```python
from build123d import *

# Parameters (mm, degrees)
F1_DEPTH = 13
F2_R     = 1
F3_DEPTH = 1.5
F4_R     = 2
F5_DEPTH = 3


with BuildPart() as f1:
    # F0 (on Top) → F1 (new body)
    with BuildSketch(Plane.XY):
        Polygon((-10.700272, 20.6891), (-33.300272, 20.6891), (-33.300272, 4.6891), (-38.300272, 4.6891), (-38.300272, 3.1891), (-33.300272, 3.1891), (-33.300272, -2.5109), (-10.700272, -2.5109), (-10.700272, 3.1891), (-5.700272, 3.1891), (-5.700272, 4.6891), (-10.700272, 4.6891), align=None)
    extrude(amount=F1_DEPTH)

    # F2 (on face) → F3 (cut, through all)
    with BuildSketch(Plane.XZ.offset(-3.1891)):
        with Locations((-36.300272, 6.5)):
            Circle(F2_R)
        with Locations((-7.700272, 6.5)):
            Circle(F2_R)
    extrude(amount=-F3_DEPTH, mode=Mode.SUBTRACT)

    # F4 (on face) → F5 (join)
    with BuildSketch(Plane.XZ.offset(2.5109)):
        with Locations((-16.700272, 6.5)):
            Circle(F4_R)
    extrude(amount=F5_DEPTH)


solid = f1.part
```
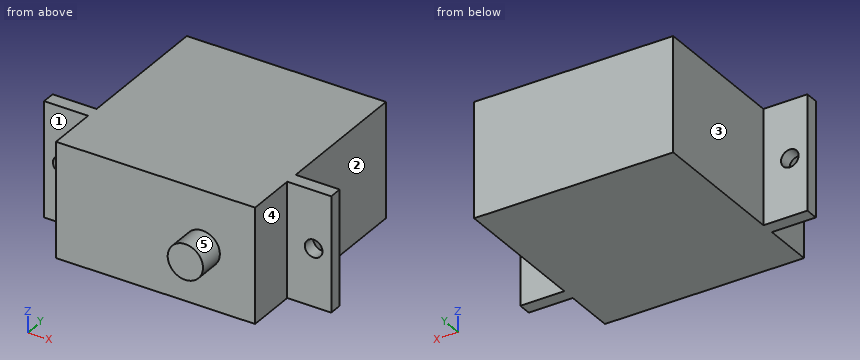
Could you check a few things on this model? Use its own coordinates, in mm. Face numbers are marked on the shaded views. A direction names the side the tool comes from. Round coordinates to 2 decimals unless told otherwise and drop trailing zeros. Loops run counter-clockwise (first coordinate to the right, second up) from the corner with the lowest first, then second, coordinate; pieces in that order, holes last. Notation, with made-up numbers: (15.5, -7.5) - (42.5, -7.5) arc R33 ccw to (42.5, 21.5) - close; hole circle Ø4 at (-38.75, -40). An arc over 180 degrees is marked (long way). Answer in a Markdown table with one row per item. Add a question column.
(1) I'm going to push flat-ended pins straight in: pin 1 (1 mm diameter, centred on x = -9, z = 4.5, fed in from +Y); pin 2 (2.5 mm diameter, centred on x = -8, z = 6, fed in from -Y); pin 3 (5 mm diameter, centred on y = 13.5, z = 2, fed in from +X). Where does each tip first touch, or does it pass through?
(2) For the marked faces 1, 2, 3, 4 and 5, which set-ups out of +Z, -Z, +X, -X, +Y, -Y let a thin tool reach every point of the face, with its end or its side?
(3) If we section it at D-D (x = -28): Please give me the cut outline in (y, z), plus the area to 3 significant figures.
(4) I need wall thicknesses on line 1 along X through (y, z) = (12.5, 5); line 2 along Y through (x, z) = (-9, 12); line 3 along Y through (x, z) = (-27, 10.5). Which ranges of each line are inside material? Lowest first, please.
(5) If we section it at A-A (z = 6.5): Please give me the cut outline in (x, y).
(6) If we section it at B-B (y = -2): Please give me the cut outline in (x, z).
(7) If we section it at C-C (x = -18): Please give me the cut outline in (y, z).
Model answer:
| question | item | result |
|---|---|---|
| 1 | pin 1 | stops at y = 4.69 |
| 1 | pin 2 | stops at y = 3.19 |
| 1 | pin 3 | stops at x = -10.7 |
| 2 | face 1 | +Z, -Z, -X, -Y |
| 2 | face 2 | +Z, -Z, +X, +Y |
| 2 | face 3 | +Z, -Z, -X, +Y |
| 2 | face 4 | +Z, -Z, +X, -Y |
| 2 | face 5 | -Y |
| 3 | outline | (-2.51, 0) - (20.69, 0) - (20.69, 13) - (-2.51, 13) - close |
| 3 | area | 302 mm² |
| 4 | line 1 | x = -33.3 to -10.7 |
| 4 | line 2 | y = 3.19 to 4.69 |
| 4 | line 3 | y = -2.51 to 20.69 |
| 5 | outline | (-38.3, 3.19) - (-37.3, 3.19) - (-37.3, 4.69) - (-38.3, 4.69) - close; (-35.3, 3.19) - (-33.3, 3.19) - (-33.3, -2.51) - (-18.7, -2.51) - (-18.7, -5.51) - (-14.7, -5.51) - (-14.7, -2.51) - (-10.7, -2.51) - (-10.7, 3.19) - (-8.7, 3.19) - (-8.7, 4.69) - (-10.7, 4.69) - (-10.7, 20.69) - (-33.3, 20.69) - (-33.3, 4.69) - (-35.3, 4.69) - close; (-6.7, 3.19) - (-5.7, 3.19) - (-5.7, 4.69) - (-6.7, 4.69) - close |
| 6 | outline | (-33.3, 0) - (-10.7, 0) - (-10.7, 13) - (-33.3, 13) - close |
| 7 | outline | (-5.51, 4.98) - (-2.51, 4.98) - (-2.51, 0) - (20.69, 0) - (20.69, 13) - (-2.51, 13) - (-2.51, 8.02) - (-5.51, 8.02) - close |
